The figure shows three views and two pictorial views of one solid part (mm, origin at its lowest corner). Answer the questions. Coordinates: 2 decimals unless noted, no trailing zeros. Loops run counter-clockwise (first coordinate to the right, second up) from the corner with the lowest first, then second, coordinate; pieces in that order, holes last. Notation, with made-up numbers: (-0.5, 14) -> (28.5, 14) arc R19 ccw to (28.5, 23) -> close; hole circle Ø3 at (53.25, 72.25). An arc over 180 degrees is marked (long way). Answer as a JSON object with one key per item and string values. Group by question number.
1) Section C-C, the plane x = 20 is taken. Give the vertices of the cut face in (y, z).
2) Flat-ended cylindrical pins translate along their axes: P1, Ø4, axis at y = 50.5, z = 21, coming from the -X side; P2, Ø10, axis at y = 67, z = 15.5, coming from the -X side; P3, Ø6, axis at x = 16, z = 17, coming from the -Y side. Find the tip coordinate at first contact, or state that the pin passes through.
3) Section B-B, the plane y = 54 is taken. Give the vertices of the cut face in (x, z), plus the area to 3 significant figures.
4) Consider probe 1 along X at (y, z) = (3, 4.5); probe 2 along X at (y, z) = (24.5, 9.5); probe 3 along Y at (x, z) = (59.5, 2.25). Determine where each line is inside the solid, lowest interval first. Write a range as [from, to].
5) Section A-A, the plane z = 2.75 is taken. Give the vertices of the cut face in (x, y), plus the area to 3 significant figures.
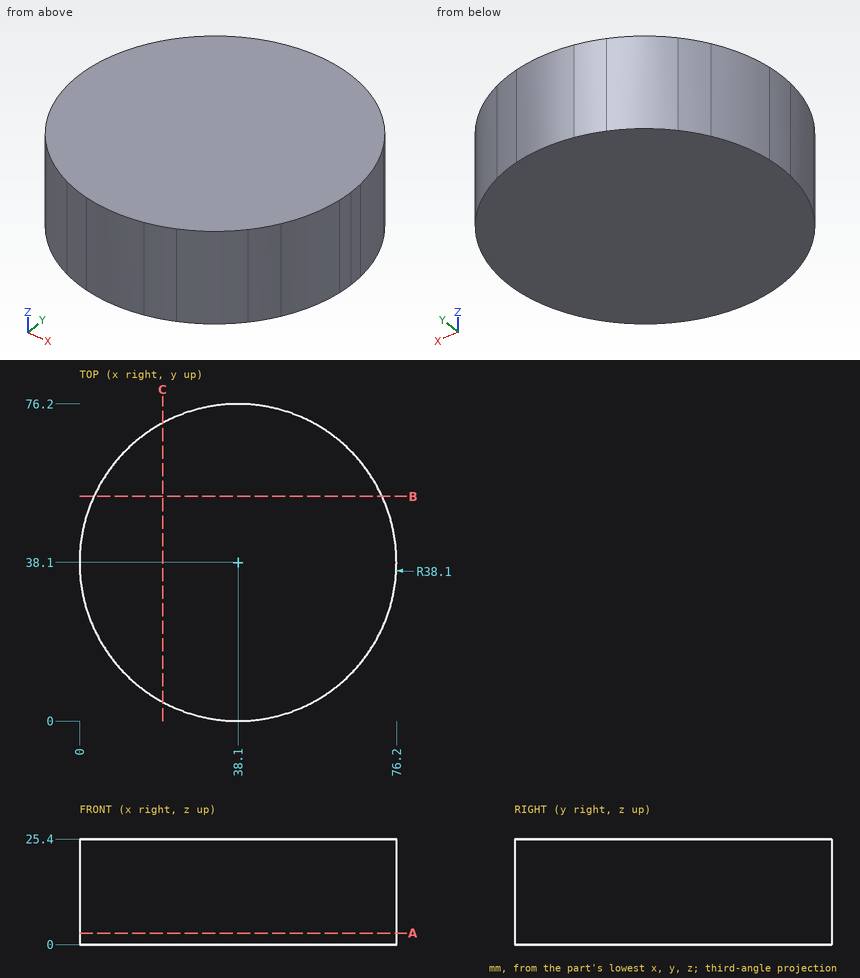
Determined:
{
 "1": {"outline": "(4.57, 0) -> (71.63, 0) -> (71.63, 25.4) -> (4.57, 25.4) -> close"},
 "2": {"P1": "x = 1.45", "P2": "x = 8.43", "P3": "y = 5.13"},
 "3": {"outline": "(3.48, 0) -> (72.72, 0) -> (72.72, 25.4) -> (3.48, 25.4) -> close", "area": "1,760 mm²"},
 "4": {"probe 1": "[23.28, 52.92]", "probe 2": "[2.51, 73.69]", "probe 3": "[6.58, 69.62]"},
 "5": {"outline": "circle Ø76.2 at (38.1, 38.1)", "area": "4,560 mm²"}
}
